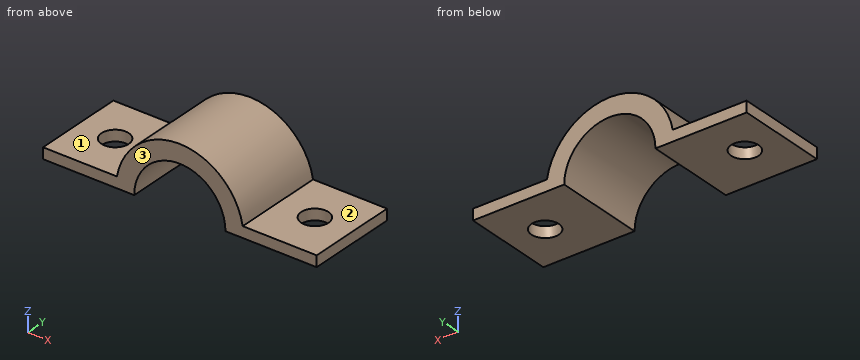
```python
from build123d import *

# Parameters (mm, degrees)
F1_DEPTH = 25
F3_D     = 7.5
F4_D     = 7.5


with BuildPart() as f1:
    # F0 (on Front) → F1 (new body)
    with BuildSketch(Plane.XZ):
        with BuildLine():
            ThreePointArc((-12.5, 0), (0, 12.5), (12.5, 0))
            Line((12.5, 0), (17.5, 0))
            Line((17.5, 0), (37.5, 0))
            Line((37.5, 0), (37.5, 3))
            Line((37.5, 3), (17.24094, 3))
            ThreePointArc((17.24094, 3), (0, 17.5), (-17.24094, 3))
            Line((-17.24094, 3), (-37.5, 3))
            Line((-37.5, 3), (-37.5, 0))
            Line((-37.5, 0), (-17.5, 0))
            Line((-17.5, 0), (-12.5, 0))
        make_face()
    extrude(amount=F1_DEPTH)

    # F3 (through all)
    with Locations(Plane.XY.offset(3)):
        with Locations((-27.37047, -12.5)):
            Hole(F3_D / 2)

    # F4 (through all)
    with Locations(Plane.XY.offset(3)):
        with Locations((27.37047, -12.5)):
            Hole(F4_D / 2)


solid = f1.part
```
CAD build for the part. Positions are in the model's coordinates, mm. Face numbers are marked on the shaded views. A direction names the side the tool comes from. Round coordinates to 2 decimals unless told otherwise and drop trailing zeros. Loops run counter-clockwise (first coordinate to the right, second up) from the corner with the lowest first, then second, coordinate; pieces in that order, holes last. Notation, with made-up numbers: M 72.25,52.25 L 101.25,52.25 A13 ccw 101.25,74.25 Z; hole C -15.75,60.25 d5. An arc over 180 degrees is marked long. Return JSON: item names as keys, results as strings. Group by question number.
(1) Drop flat-ended pins along their axis: P1, Ø8, axis at y = -15, z = 12, coming from the -X side; P2, Ø2, axis at x = -21, y = -9.5, coming from the +Z side; P3, Ø6, axis at x = 5, y = -19, coming from the -Z side; P4, Ø6, axis at x = -27.37, y = -12.5, coming from the -Z side. Give the stop position or say it passes through.
(2) Wall check: probe 1 along Z at (x, y) = (-25, -18.25); probe 2 along X at (y, z) = (-10.5, 11.5); probe 3 along X at (y, z) = (-5.25, 3.5). Give the ranges that are in metal, low to high. Write a range as [from, to].
(3) Tool access for the marked faces 1, 2 and 3: list every direction of +Z, -Z, +X, -X, +Y, -Y with a clear straight run to the whole face (end or side of a thin tool).
(4) Saw through at D-D, the plane y = -7.75. List the corners of the cut face in (x, z).
(5) Saw through at C-C, the plane x = 28.5. List the corners of the cut face in (y, z).
(6) Saw through at A-A, the plane y = -12.5. List the corners of the cut face in (x, z).
(7) Saw through at B-B, the plane z = 7.25. List the corners of the cut face in (x, y).
Answer list:
{
 "1": {"P1": "x = -15.56", "P2": "z = 3", "P3": "z = 9.6", "P4": "through"},
 "2": {"probe 1": "[0, 3]", "probe 2": "[-13.19, -4.9], [4.9, 13.19]", "probe 3": "[-17.15, -12], [12, 17.15]"},
 "3": {"face 1": "+Z, -X, +Y, -Y", "face 2": "+Z, +X, +Y, -Y", "face 3": "+Z, -Z, +X, -X, -Y"},
 "4": {"outline": "M -37.5,0 L -12.5,0 A12.5 cw 12.5,0 L 37.5,0 L 37.5,3 L 17.24,3 A17.5 ccw -17.24,3 L -37.5,3 Z"},
 "5": {"outline": "M -25,0 L -16.08,0 L -16.08,3 L -25,3 Z; M -8.92,0 L 0,0 L 0,3 L -8.92,3 Z"},
 "6": {"outline": "M -37.5,0 L -31.12,0 L -31.12,3 L -37.5,3 Z; M -23.62,0 L -12.5,0 A12.5 cw 12.5,0 L 23.62,0 L 23.62,3 L 17.24,3 A17.5 ccw -17.24,3 L -23.62,3 Z; M 31.12,0 L 37.5,0 L 37.5,3 L 31.12,3 Z"},
 "7": {"outline": "M -15.93,-25 L -10.18,-25 L -10.18,0 L -15.93,0 Z; M 10.18,-25 L 15.93,-25 L 15.93,0 L 10.18,0 Z"}
}
